Here's how the part is built. I have some questions about the finished solid (model axes, mm). A direction names the side the tool comes from. Coordinates: 2 decimals unless noted, no trailing zeros. Order: outer loops, then holes, each group sorted by start corner. A loop starts at its lowest first (then second) coordinate and runs counter-clockwise, first axis right, second up. Notation, with made-up numbers: M 12.25,58 L 24.25,58 A28 cw 24.25,79 Z; hole C 50,5 d6. An arc over 180 degrees is marked long. One line per question, with ' | ' between items. Start each with the question number.
```python
from build123d import *

# Parameters (mm, degrees)
F0_W     = 31.75
F0_H     = 76.2
F1_DEPTH = 19.05
F0_W_2   = 57.15
F2_DEPTH = 6.35
F3_R     = 6.35
F4_DEPTH = 15.24
F5_W     = 10.541
F5_H     = 52.705
F5_H_2   = 39.37
F6_DEPTH = 1.905
F7_DEPTH = 1.27


with BuildPart() as f1:
    # F0 (on Top) → F1 (new body)
    with BuildSketch(Plane.XY):
        with Locations((-24.9883290738, -11.122222997)):
            Rectangle(F0_W, F0_H)
    extrude(amount=F1_DEPTH)

    # F0 (on Top) → F2 (join)
    with BuildSketch(Plane.XY):
        with Locations((19.4616709262, -11.122222997)):
            Rectangle(F0_W_2, F0_H)
        with Locations((-24.9883290738, -11.122222997)):
            Rectangle(F0_W, F0_H)
    extrude(amount=F2_DEPTH)

    # F3 (on face) → F4 (cut)
    with BuildSketch(Plane.XY.offset(19.05)):
        with Locations((-33.2433290738, 14.277777003)):
            Circle(F3_R)
        with Locations((-16.7333290738, 14.277777003)):
            Circle(F3_R)
        with Locations((-33.2433290738, -11.122222997)):
            Circle(F3_R)
        with Locations((-16.7333290738, -11.122222997)):
            Circle(F3_R)
        with Locations((-16.7333290738, -36.522222997)):
            Circle(F3_R)
        with Locations((-33.2433290738, -36.522222997)):
            Circle(F3_R)
    extrude(amount=-F4_DEPTH, mode=Mode.SUBTRACT)

    # F5 (on face) → F6 (cut)
    with BuildSketch(Plane.XY.offset(6.35)):
        with Locations((12.4131709262, -1.914722997)):
            Rectangle(F5_W, F5_H)
        with Locations((-1.3028290738, -1.914722997)):
            Rectangle(F5_W, F5_H)
        with Locations((39.8451709262, 4.752777003)):
            Rectangle(F5_W, F5_H_2)
        with Locations((26.1291709262, -1.914722997)):
            Rectangle(F5_W, F5_H)
        Polygon((32.0029154061, -35.6534661021), (-3.5570845939, -35.6534661021), (-3.5570845939, -43.0194661021), (12.9529154061, -43.0194661021), (12.9529154061, -41.4954661021), (32.0029154061, -41.4954661021), align=None)
    extrude(amount=-F6_DEPTH, mode=Mode.SUBTRACT)

    # F7 (add): a face of the model
    f7_faces = [f1.faces().sort_by_distance(p)[0] for p in [
        (13.1938987856, -38.9723525287, 4.445),
    ]]
    extrude(f7_faces, amount=F7_DEPTH)


solid = f1.part
```
1. Imagine slicing it at C-C (z = 16.75). List the corners of the cut face in (x, y) for me.
2. Which directions (+Z, -Z, +X, -X, +Y, -Y) give clear straight access to the entire face, cutting with the end or side of a thin tool? Please do faces 3 (the face through (19, -19, 6.35)), 4 (the face through (26, 24.438, 5)).
3. Imagine slicing it at A-A (y = -1). List the corners of the cut face in (x, z) for me (3 decimals).
4. Will these pins go through, and if not, where does the flat tip stop? pin 1 (8.5 mm diameter, centred on x = 39, y = 4, fed in from +Z) (3 decimals); pin 2 (10 mm diameter, centred on x = -33, y = -36.5, fed in from +Z); pin 3 (8 mm diameter, centred on x = 19, y = -39, fed in from -Z); pin 4 (1 mm diameter, centred on y = 6.5, z = 15, fed in from +X).
5. We'd pull the mould along Y, two halves only. Please class faces 1 (the face through (-6.573, -2, 5)), 2 (the face through (3, -11, 0)): released by +Y, released by -Y, zero draft, split by the parting line, or undercut.
6. I need wall thicknesses on line 1 (X direction, y = 14, z = 17.75); line 2 (Y direction, x = -36.5, z = 4.5); line 3 (X direction, y = 12, z = 13.75). Which ranges of each line are inside material? Lowest first, please.
7. Imagine slicing it at B-B (x = 25.5). List the corners of the cut face in (y, z) for me (3 decimals), then the cut area to 3 significant figures.
8. Imagine slicing it at D-D (x = 2). List the corners of the cut face in (y, z) for me (3 decimals).
Entries:
1) outline: M -40.86,-49.22 L -9.11,-49.22 L -9.11,26.98 L -40.86,26.98 Z; hole C -33.24,-36.52 d12.7; hole C -33.24,-11.12 d12.7; hole C -33.24,14.28 d12.7; hole C -16.73,-36.52 d12.7; hole C -16.73,-11.12 d12.7; hole C -16.73,14.28 d12.7
2) face 3: +Z, +X, +Y, -Y | face 4: +Z
3) outline: M -40.863,0 L 48.037,0 L 48.037,6.35 L 45.116,6.35 L 45.116,4.445 L 34.575,4.445 L 34.575,6.35 L 31.4,6.35 L 31.4,4.445 L 20.859,4.445 L 20.859,6.35 L 17.684,6.35 L 17.684,4.445 L 7.143,4.445 L 7.143,6.35 L 3.968,6.35 L 3.968,4.445 L -6.573,4.445 L -6.573,6.35 L -9.113,6.35 L -9.113,19.05 L -40.863,19.05 Z
4) pin 1: z = 4.445 | pin 2: z = 3.81 | pin 3: z = 0 | pin 4: x = -9.11
5) face 1: undercut | face 2: zero draft
6) line 1: -40.86 to -39.59, -26.9 to -23.08, -10.39 to -9.11 | line 2: -49.22 to -41.97, -31.07 to -16.57, -5.67 to 8.83, 19.73 to 26.98 | line 3: -40.86 to -39.17, -27.32 to -22.66, -10.81 to -9.11
7) outline: M -49.222,0 L 26.978,0 L 26.978,6.35 L 24.438,6.35 L 24.438,4.445 L -28.267,4.445 L -28.267,6.35 L -35.653,6.35 L -35.653,5.715 L -41.495,5.715 L -41.495,6.35 L -49.222,6.35 Z | area: 380 mm²
8) outline: M -49.222,0 L 26.978,0 L 26.978,6.35 L 24.438,6.35 L 24.438,4.445 L -28.267,4.445 L -28.267,6.35 L -35.653,6.35 L -35.653,5.715 L -43.019,5.715 L -43.019,6.35 L -49.222,6.35 Z
